from build123d import *

# Parameters (mm, degrees)
F0_W     = 12.7
F0_H     = 63.5
F1_DEPTH = 63.5
F2_DEPTH = 63.5
F3_T     = -12.7


with BuildPart() as f1:
    # F0 (on Front) → F1 (new body)
    with BuildSketch(Plane.XZ):
        with Locations((6.35, -31.75)):
            Rectangle(F0_W, F0_H)
    extrude(amount=F1_DEPTH)

    # F2 (add): a face of the model
    f2_faces = [f1.faces().sort_by_distance(p)[0] for p in [
        (12.7, -31.75, -31.75),
    ]]
    extrude(f2_faces, amount=F2_DEPTH)

    # F3
    f3_openings = [f1.faces().sort_by_distance(p)[0] for p in [
        (38.1, -63.5, -31.75),
        (38.1, -31.75, 0),
        (76.2, -31.75, -31.75),
    ]]
    offset(amount=F3_T, openings=f3_openings)


solid = f1.part
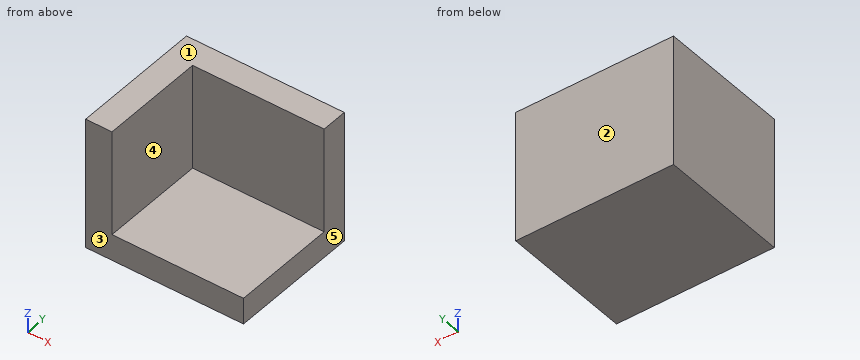
The listing builds one solid part. Answer for the finished solid, in the listing's coordinates (mm). Face numbers are marked on the shaded views. A direction names the side the tool comes from. Coordinates: 2 decimals unless noted, no trailing zeros. Order: outer loops, then holes, each group sorted by start corner. A loop starts at its lowest first (then second) coordinate and runs counter-clockwise, first axis right, second up. Notation, with made-up numbers: M -8,76 L -3,76 A23 ccw -3,89 Z; hole C 50.25,89 d4. An arc over 180 degrees is marked long. Use CSV: the item, a comma, the result in double quotes.
Q1. A tool of negligible diameter and unlimited length cuts with its end or side. For the marked faces 4 and 5, from which of +Z, -Z, +X, -X, +Y, -Y can it reach the whole face along a straight path? Write none if from no direction.
Here are the results:
face 4,"+Z, +X, -Y"
face 5,"+Z, -Z, +X, +Y, -Y"
Q2. Given pin 1 Ø2 at (x, z) = (26.5, -54) entering from +Y; pin 2 Ø15 at (x, y) = (30.5, -27) entering from +Z; pin 3 Ø8 at (x, z) = (19, -22) entering from -Y, each flat-ended and moving along its own axis, determine where each tip first touches the part or whether it passes through.
Here are the results:
pin 1,"y = 0"
pin 2,"z = -50.8"
pin 3,"y = -12.7"
Q3. Straight lines are drawn through the part: L1, parallel to X at y = -22.5, z = -36; L2, parallel to Z at x = 57, y = -19; L3, parallel to Y at x = 41.5, z = -43.5. For each, find the intervals that lie inside material, in ascending order.
Here are the results:
L1,"0 to 12.7"
L2,"-63.5 to -50.8"
L3,"-12.7 to 0"
Q4. Section A-A (y = -47.5) is taken. Determine the outline of the cut face in (x, z), then the cut area to 3 significant figures.
Here are the results:
outline,"M 0,-63.5 L 76.2,-63.5 L 76.2,-50.8 L 12.7,-50.8 L 12.7,0 L 0,0 Z"
area,"1,610 mm2"
Q5. Section B-B (x = 21.5) is taken. Determine the outline of the cut face in (y, z), then the cut area to 3 significant figures.
Here are the results:
outline,"M -63.5,-63.5 L 0,-63.5 L 0,0 L -12.7,0 L -12.7,-50.8 L -63.5,-50.8 Z"
area,"1,450 mm2"
Q6. Determine the mould class of the marked faces 1, 2 and 3 for opening direction Y: pulls with the +Y half, pulls with the -Y half, needs draft (parallel to the pull), parting line crosses it, or undercut.
Here are the results:
face 1,"needs draft"
face 2,"pulls with the +Y half"
face 3,"pulls with the -Y half"
